Answer from the drawing. Dimensions are ordinates in mm from the lowest x, y and z of the part. Round coordinates to 2 decimals unless told otherwise and drop trailing zeros. Loops run counter-clockwise (first coordinate to the right, second up) from the corner with the lowest first, then second, coordinate; pieces in that order, holes last. Notation, with made-up numbers: (-1, -37) - (49, -37) arc R10 ccw to (49, -28) - close; hole circle Ø9 at (-23, 60). An arc over 180 degrees is marked (long way). Write item = value, one per line. Start each with the question number.
1) Section D-D, the plane z = 11.75 is taken. Determine the outline of the cut face in (x, y), and give its area (3 significant figures).
2) Given pin 1 Ø2.5 at (y, z) = (97.5, 21.5) entering from -X; pin 2 Ø1.5 at (x, y) = (108.5, 20) entering from -Z; pin 3 Ø1.5 at (x, z) = (31, 19.5) entering from +Y; pin 4 Ø8 at (y, z) = (138, 12.5) entering from +X, each flat-ended and moving along its own axis, determine where each tip first touches the part or whether it passes through.
3) Section A-A, the plane x = 59.5 is taken. Determine the outline of the cut face in (y, z), and give its area (3 significant figures).
4) Section C-C, the plane x = 90 is taken. Determine the outline of the cut face in (y, z).
5) Straight lines are drawn through the part: line 1 along Y through (x, z) = (56, 19.25); line 2 along X through (y, z) = (124.5, 18.25); line 3 along Z through (x, y) = (121.5, 78). For each, find the intervals that lie inside material, in ascending order.
6) Section B-B, the plane y = 104.5 is taken. Determine the outline of the cut face in (x, z).
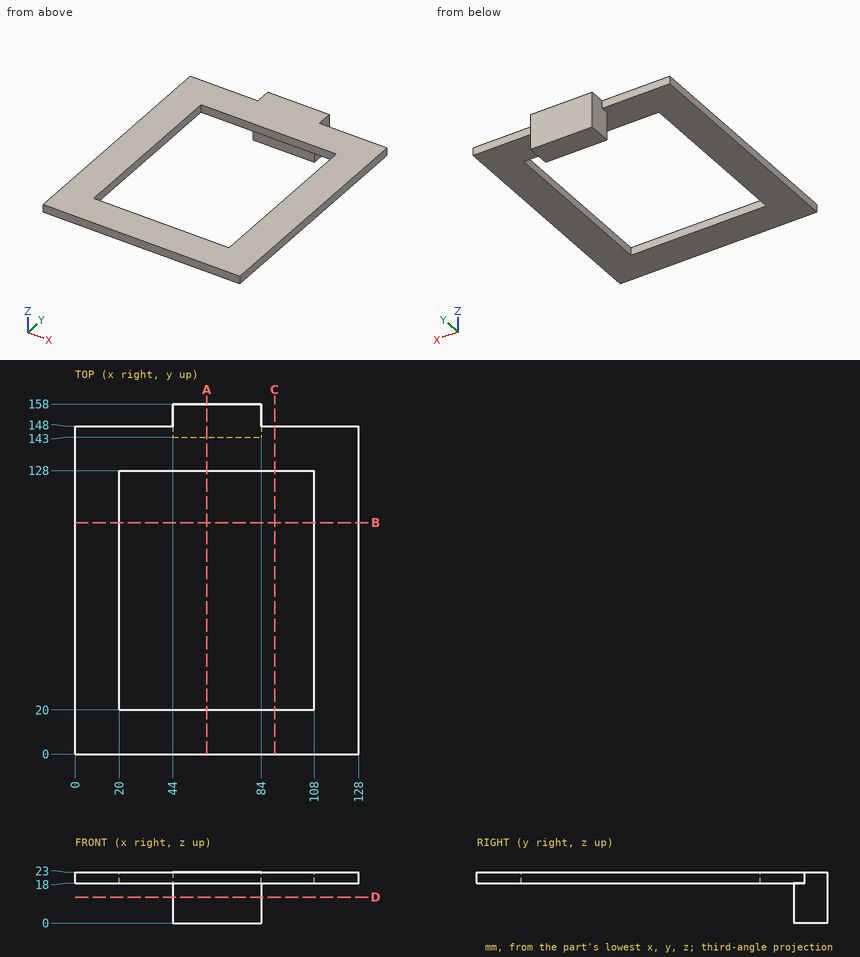
Geometry check:
q1.outline = (44, 143) - (84, 143) - (84, 158) - (44, 158) - close
q1.area = 600 mm2
q2.pin_1 = 0
q2.pin_2 = 18
q2.pin_3 = 148
q2.pin_4 = through
q3.outline = (0, 18) - (20, 18) - (20, 23) - (0, 23) - close; (128, 18) - (143, 18) - (143, 0) - (158, 0) - (158, 23) - (128, 23) - close
q3.area = 520 mm2
q4.outline = (0, 18) - (20, 18) - (20, 23) - (0, 23) - close; (128, 18) - (148, 18) - (148, 23) - (128, 23) - close
q5.line_1 = 0 to 20, 128 to 158
q5.line_2 = 0 to 20, 108 to 128
q5.line_3 = 18 to 23
q6.outline = (0, 18) - (20, 18) - (20, 23) - (0, 23) - close; (108, 18) - (128, 18) - (128, 23) - (108, 23) - close
